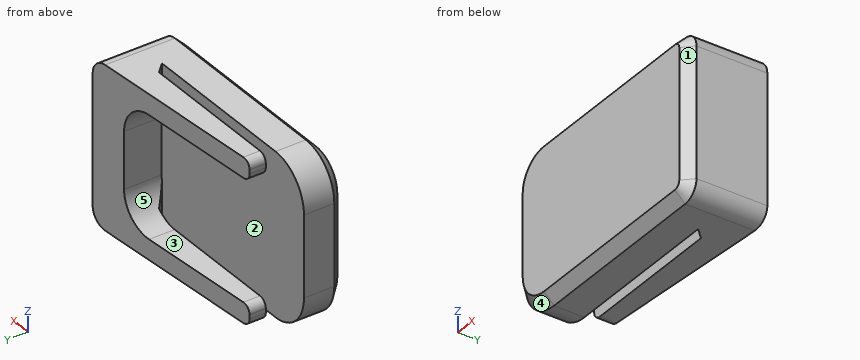
from build123d import *

# Parameters (mm, degrees)
BOSS_EXTRUDE1_DEPTH = 12.7
SKETCH2_W           = 19.05
SKETCH2_H           = 6.35
CUT_EXTRUDE1_DEPTH  = 31.75
CUT_EXTRUDE2_DEPTH  = 35.195796525
CHAMFER3_SIZE       = 1.5875
FILLET1_R           = 1.27
FILLET2_R           = 5.08


with BuildPart() as part:
    # Sketch1 → Boss-Extrude1 (new body)
    with BuildSketch(Plane(origin=(0, 0, 0), x_dir=(1, 0, 0), z_dir=(0, 1, 0))):
        with BuildLine():
            Line((-12.7, -12.7), (16.51, -12.7))
            ThreePointArc((16.51, -12.7), (18.306051224, -11.956051224), (19.05, -10.16))
            Line((19.05, -10.16), (19.05, 10.16))
            ThreePointArc((19.05, 10.16), (18.306051224, 11.956051224), (16.51, 12.7))
            Line((16.51, 12.7), (-12.7, 12.7))
            ThreePointArc((-12.7, 12.7), (-17.190128061, 10.840128061), (-19.05, 6.35))
            Line((-19.05, 6.35), (-19.05, -6.35))
            ThreePointArc((-19.05, -6.35), (-17.190128061, -10.840128061), (-12.7, -12.7))
        make_face()
    extrude(amount=BOSS_EXTRUDE1_DEPTH)

    # Sketch2 → Cut-Extrude1 (cut)
    with BuildSketch(Plane.ZY.offset(19.05)):
        with Locations((0, 9.525)):
            Rectangle(SKETCH2_W, SKETCH2_H)
    extrude(amount=-CUT_EXTRUDE1_DEPTH, mode=Mode.SUBTRACT)

    # Sketch3 → Cut-Extrude2 (cut, through all)
    with BuildSketch(Plane.XY.offset(12.7)):
        Polygon((19.05, 12.7), (-19.05, 12.7), (-19.05, 6.35), (12.065, 6.35), (12.7, 6.35), (12.7, 6.985), (12.7, 7.239), (12.7, 7.874), (12.065, 7.874), (-12.7, 7.874), (-12.7, 10.414), align=None)
    extrude(amount=-CUT_EXTRUDE2_DEPTH, mode=Mode.SUBTRACT)

    # Chamfer3
    # the kernel refuses this chamfer: 1.5875 mm, written as the material it adds along each edge
    with BuildSketch(Plane(origin=(12.7, 7.874, 12.7), x_dir=(0.027495876610588915, -0.9996219169112966, 0), z_dir=(0, 0, -1))) as chamfer3_piece_1:
        Polygon((CHAMFER3_SIZE * 0.999621916911, CHAMFER3_SIZE * 0.0274958766106), (-CHAMFER3_SIZE * 0.0274958766106, CHAMFER3_SIZE * 0.999621916911), (0, 0), align=None)
    extrude(amount=3.175)
    with BuildSketch(Plane(origin=(12.7, 7.874, -9.525), x_dir=(-0.9996219169112968, 0.027495876610586185, 0), z_dir=(0, 0, -1))) as chamfer3_piece_2:
        Polygon((CHAMFER3_SIZE * 0.999621916911, -CHAMFER3_SIZE * 0.0274958766106), (-CHAMFER3_SIZE * 0.0274958766106, -CHAMFER3_SIZE * 0.999621916911), (0, 0), align=None)
    extrude(amount=3.175)
    # the kernel refuses this chamfer: 1.5875 mm, written as the material it takes off along each edge
    with BuildSketch(Plane(origin=(-12.7, 0, 12.7), x_dir=(0, 0.9996219169112966, 0.027495876610586743), z_dir=(1, 0, 0)), Plane(origin=(16.51, 0, -12.7), x_dir=(0, 0.9996219169112966, -0.027495876610586743), z_dir=(-1, 0, 0))) as chamfer3_2_piece_1:
        Polygon((CHAMFER3_SIZE * 0.999621916911, -CHAMFER3_SIZE * 0.0274958766106), (-CHAMFER3_SIZE * 0.0274958766106, -CHAMFER3_SIZE * 0.999621916911), (0, 0), align=None)
    extrude(amount=29.21, mode=Mode.SUBTRACT)
    with BuildSketch(Plane(origin=(16.51, 0, 10.16), x_dir=(0, 0, 1), z_dir=(-1, 0, 0))) as chamfer3_2_piece_2:
        Polygon((2.54 - CHAMFER3_SIZE, 0), (2.54, CHAMFER3_SIZE), (2.54, 0), align=None)
    revolve(axis=Axis((16.51, 0, 10.16), (0, 1, 0)), revolution_arc=90, mode=Mode.SUBTRACT)
    with BuildSketch(Plane(origin=(19.05, 0, 10.16), x_dir=(0.027495876610585654, 0.9996219169112966, 0), z_dir=(0, 0, -1))) as chamfer3_2_piece_3:
        Polygon((CHAMFER3_SIZE * 0.999621916911, -CHAMFER3_SIZE * 0.0274958766106), (-CHAMFER3_SIZE * 0.0274958766106, -CHAMFER3_SIZE * 0.999621916911), (0, 0), align=None)
    extrude(amount=20.32, mode=Mode.SUBTRACT)
    with BuildSketch(Plane(origin=(16.51, 0, -10.16), x_dir=(1, 0, 0), z_dir=(0, 0, 1))) as chamfer3_2_piece_4:
        Polygon((2.54, CHAMFER3_SIZE), (2.54 - CHAMFER3_SIZE, 0), (2.54, 0), align=None)
    revolve(axis=Axis((16.51, 0, -10.16), (0, 1, 0)), revolution_arc=90, mode=Mode.SUBTRACT)
    with BuildSketch(Plane(origin=(-12.7, 0, -6.35), x_dir=(0, 0, -1), z_dir=(1, 0, 0))) as chamfer3_2_piece_5:
        Polygon((6.35, CHAMFER3_SIZE), (6.35 - CHAMFER3_SIZE, 0), (6.35, 0), align=None)
    revolve(axis=Axis((-12.7, 0, -6.35), (0, 1, 0)), revolution_arc=90, mode=Mode.SUBTRACT)
    with BuildSketch(Plane(origin=(-12.7, 0, 6.35), x_dir=(-1, 0, 0), z_dir=(0, 0, -1))) as chamfer3_2_piece_6:
        Polygon((6.35, CHAMFER3_SIZE), (6.35 - CHAMFER3_SIZE, 0), (6.35, 0), align=None)
    revolve(axis=Axis((-12.7, 0, 6.35), (0, 1, 0)), revolution_arc=90, mode=Mode.SUBTRACT)
    with BuildSketch(Plane(origin=(-19.05, 0, -6.35), x_dir=(-0.027495876610585654, 0.9996219169112966, 0), z_dir=(0, 0, 1))) as chamfer3_2_piece_7:
        Polygon((CHAMFER3_SIZE * 0.999621916911, -CHAMFER3_SIZE * 0.0274958766106), (-CHAMFER3_SIZE * 0.0274958766106, -CHAMFER3_SIZE * 0.999621916911), (0, 0), align=None)
    extrude(amount=12.7, mode=Mode.SUBTRACT)

    # Fillet1
    fillet1_edges = [part.edges().sort_by_distance(p)[0] for p in [
        (-12.7, 9.144, -9.525),
        (-12.7, 9.144, 9.525),
        (-12.7, 9.144, -12.7),
        (-12.7, 9.144, 12.7),
    ]]
    fillet(fillet1_edges, radius=FILLET1_R)

    # Fillet2
    fillet2_edges = [part.edges().sort_by_distance(p)[0] for p in [
        (12.7, 9.2964, -9.525),
        (12.7, 9.2964, 9.525),
    ]]
    fillet(fillet2_edges, radius=FILLET2_R)


solid = part.part
Can you work these out from the model? Positions are in its coordinate system, mm. Face numbers are marked on the shaded views. A direction names the side the tool comes from. Round coordinates to 2 decimals unless told otherwise and drop trailing zeros. Write each loop counter-clockwise with the first axis right and the second up, starting at its lowest first coordinate (ties: lowest second). Pieces come first, ordered by that corner, then holes. Notation, with made-up numbers: (5, 73.25) -> (60, 73.25) arc R11 ccw to (60, 92.25) -> close; hole circle Ø5 at (-21.5, 15). An arc over 180 degrees is marked (long way). Use one line per item in the form item = value. Start each with the question number.
Q1. If I drill on probe 1 along Z at (x, y) = (-10, 8.5) (3 decimals); probe 2 along Y at (x, z) = (-1.5, 4); probe 3 along Z at (x, y) = (-12, 9.25), over which ranges is the centre line in solid material (lowest first)? Write a range as [from, to].
Q2. We'd pull the mould along Y, two halves only. Please class the marked faces 1, 2 and 3: +Y half, -Y half, draft (parallel to the pull), parting line (faces both ways), or undercut.
Q3. Which directions (+Z, -Z, +X, -X, +Y, -Y) give clear straight access to the entire face, cutting with the end or side of a thin tool? Please do the marked faces 4 and 5.
Q4. Imagine slicing it at A-A (x = -3.5). Count the separate pieces of the cut face and the enclosed holes in it, then the cut area to 3 significant figures.
Q5. Imagine slicing it at D-D (y = 9.75). Please give me the cut outline in (x, z) (3 decimals).
Q6. Imagine slicing it at C-C (z = -2.25). Please give me the cut outline in (x, y), then the cut area to 3 significant figures.
Q7. Imagine slicing it at B-B (y = 3.25). Please give me the cut outline in (x, z).
Q8. I'm going to push flat-ended pins straight in: P1, Ø0.7, axis at y = 8.5, z = 11, coming from the -X side; P2, Ø5, axis at x = 6.5, z = 1, coming from the +Y side; P3, Ø10, axis at x = 14.5, z = -4.5, coming from the +Y side. Where does each tip first touch, or does it pass through?
Worked out:
q1.probe_1 = [-12.7, -9.525], [9.525, 12.7]
q1.probe_2 = [0, 6.35]
q1.probe_3 = [-12.56, -9.66], [9.66, 12.56]
q2.face_1 = -Y half
q2.face_2 = undercut
q2.face_3 = draft
q3.face_4 = -Z, -X, -Y
q3.face_5 = -X, +Y
q4.separate_pieces = 3
q4.enclosed_holes = 0
q4.area = 179 mm^2
q5.outline = (-12.7, -11.43) arc R1.27 ccw to (-11.43, -12.7) -> (16.51, -12.7) arc R2.54 ccw to (19.05, -10.16) -> (19.05, 10.16) arc R2.54 ccw to (16.51, 12.7) -> (-11.43, 12.7) arc R1.27 ccw to (-12.7, 11.43) -> (-12.7, 10.795) arc R1.27 ccw to (-11.43, 9.525) -> (7.62, 9.525) arc R5.08 cw to (12.7, 4.445) -> (12.7, -4.445) arc R5.08 cw to (7.62, -9.525) -> (-11.43, -9.525) arc R1.27 ccw to (-12.7, -10.795) -> close
q6.outline = (-19.05, 1.59) -> (-17.46, 0) -> (17.46, 0) -> (19.05, 1.59) -> (19.05, 12.7) -> (12.7, 12.24) -> (12.7, 6.35) -> (-19.05, 6.35) -> close
q6.area = 278 mm^2
q7.outline = (-19.05, -6.35) arc R6.35 ccw to (-12.7, -12.7) -> (16.51, -12.7) arc R2.54 ccw to (19.05, -10.16) -> (19.05, 10.16) arc R2.54 ccw to (16.51, 12.7) -> (-12.7, 12.7) arc R6.35 ccw to (-19.05, 6.35) -> close
q8.P1 = -12.7
q8.P2 = 6.35
q8.P3 = 12.7
